CAD build for the part. Positions are in the model's coordinates, mm. A direction names the side the tool comes from. Coordinates: 2 decimals unless noted, no trailing zeros. Loops run counter-clockwise (first coordinate to the right, second up) from the corner with the lowest first, then second, coordinate; pieces in that order, holes last. Notation, with made-up numbers: (58, -8.5) -> (98, -8.5) arc R17 cw to (98, 11.5) -> close; hole circle Ø1 at (27.5, 35.25). An arc over 180 degrees is marked (long way). Write each question's results on one line, items separated by ' | '.
Autodesk Inventor part; units mm, degrees
ref_plane "YZ Plane" through (0, 0, 0) normal (1, 0, 0) x (0, 1, 0)
ref_plane "XZ Plane" through (0, 0, 0) normal (0, 1, 0) x (-1, 0, 0)
ref_plane "XY Plane" through (0, 0, 0) normal (0, 0, 1) x (1, 0, 0)
sketch "Sketch1" plane through (0, 0, 0) normal (0, 0, 1) x (1, 0, 0)
  line L0 (-134, -130.1931) -> (134, -130.1931)
  line L1 (134, -130.1931) -> (134, 130.1931)
  line L2 (134, 130.1931) -> (-134, 130.1931)
  line L3 (-134, 130.1931) -> (-134, -130.1931)
  line L4 (-134, -130.1931) -> (134, 130.1931) construction
  line L5 (134, -130.1931) -> (-134, 130.1931) construction
  point P0 (0, 0)
  dimension "d0" = 268
  dimension "d1" = 260.3863
extrude "Extrusion1" add sketch "Sketch1" along normal blind 6
sketch "Sketch2" plane through (0, 0, 6) normal (0, 0, 1) x (1, 0, 0)
  line L0 (-134, -130.1931) -> (134, -130.1931)
  line L1 (134, 130.1931) -> (-134, 130.1931)
  line L2 (-134, 130.1931) -> (-134, -130.1931)
  line L3 (-131.125, 122.1931) -> (-124.875, 122.1931)
  line L4 (-124.875, 122.1931) -> (-124.875, -122.1931)
  line L5 (-124.875, -122.1931) -> (-131.125, -122.1931)
  line L6 (-131.125, -122.1931) -> (-131.125, 122.1931)
  line L7 (-131.125, 122.1931) -> (-124.875, -122.1931) construction
  line L8 (-124.875, 122.1931) -> (-131.125, -122.1931) construction
  point P0 (0, 0)
  point P1 (-128, 0)
  dimension "d5" = 2.875
  dimension "d6" = 6.25
  dimension "d7" = 8
  dimension "d101" = 8
extrude "Extrusion2" cut sketch "Sketch2" against normal through all
mirror "Mirror1" about plane through (0, 0, 0) normal (1, 0, 0) of "Extrusion2"
fillet "Fillet1" radius 3 4 edges at (134, 130.1931, 3) (134, -130.1931, 3) (-134, 130.1931, 3) (-134, -130.1931, 3)
sketch "Sketch3" plane through (0, 0, 6) normal (0, 0, 1) x (1, 0, 0)
  line L0 (131, 130.1931) -> (-131, 130.1931)
  line L1 (-124.875, 122.1931) -> (-124.875, -122.1931)
  line L2 (-104.875, -110.1931) -> (104.875, -110.1931)
  line L3 (104.875, -110.1931) -> (104.875, 110.1931)
  line L4 (104.875, 110.1931) -> (-104.875, 110.1931)
  line L5 (-104.875, 110.1931) -> (-104.875, -110.1931)
  line L6 (-104.875, -110.1931) -> (104.875, 110.1931) construction
  line L7 (104.875, -110.1931) -> (-104.875, 110.1931) construction
  point P0 (0, 0)
  dimension "d12" = 20
  dimension "d13" = 20
extrude "Extrusion3" cut sketch "Sketch3" against normal through all
properties part number "TopDiagonalPanel"
1) Slice it at A-A (z = 3.75). Write the cut outline in (x, y) (3 decimals).
Outcome:
outline: (-134, -127.193) arc R3 ccw to (-131, -130.193) -> (131, -130.193) arc R3 ccw to (134, -127.193) -> (134, 127.193) arc R3 ccw to (131, 130.193) -> (-131, 130.193) arc R3 ccw to (-134, 127.193) -> close; hole (-131.125, -122.193) -> (-124.875, -122.193) -> (-124.875, 122.193) -> (-131.125, 122.193) -> close; hole (-104.875, -110.193) -> (104.875, -110.193) -> (104.875, 110.193) -> (-104.875, 110.193) -> close; hole (124.875, -122.193) -> (131.125, -122.193) -> (131.125, 122.193) -> (124.875, 122.193) -> close
2) Two-plate mould, pull along Y, no slides. Class faces 3 (the flat face through (-2, -130.193, 3)), 4 (the flat face through (131.125, 2, 3)), 5 (the flat face through (134, -2, 3)), 6 (the flat face through (2, 130.193, 3)): pulls with the +Y half, pulls with the -Y half, needs draft (parallel to the pull), parting line crosses it, or undercut.
Outcome:
face 3: pulls with the -Y half | face 4: undercut | face 5: needs draft | face 6: pulls with the +Y half
3) Slice it at B-B (y = -58). Write the cut outline in (x, z) (3 decimals), then the cut area to 4 significant figures.
Outcome:
outline: (-134, 0) -> (-131.125, 0) -> (-131.125, 6) -> (-134, 6) -> close; (-124.875, 0) -> (-104.875, 0) -> (-104.875, 6) -> (-124.875, 6) -> close; (104.875, 0) -> (124.875, 0) -> (124.875, 6) -> (104.875, 6) -> close; (131.125, 0) -> (134, 0) -> (134, 6) -> (131.125, 6) -> close | area: 274.5 mm^2
4) Which spindle directions (+Z, -Z, +X, -X, +Y, -Y) get a long thin tool onto all of the face, cutting with end or side? Do faces 1 (the flat face through (124.875, -2, 3)), 2 (the flat face through (-134, 2, 3)). Say none if no direction does.
Outcome:
face 1: +Z, -Z | face 2: +Z, -Z, -X, +Y, -Y
5) Slice it at C-C (x = -57). Write the cut outline in (y, z).
Outcome:
outline: (-130.19, 0) -> (-110.19, 0) -> (-110.19, 6) -> (-130.19, 6) -> close; (110.19, 0) -> (130.19, 0) -> (130.19, 6) -> (110.19, 6) -> close
6) Drill centre lines: L1, parallel to X at y = 11, z = 0.35 (3 decimals); L2, parallel to Y at x = -10, z = 5.1. Where is each one in solid material? Low to high. Write a range as from..to.
Outcome:
L1: x = -134..-131.125, -124.875..-104.875, 104.875..124.875, 131.125..134 | L2: y = -130.19..-110.19, 110.19..130.19
